CAD build for the part. Positions are in the model's coordinates, mm. A direction names the side the tool comes from. Round coordinates to 2 decimals unless told otherwise and drop trailing zeros. Loops run counter-clockwise (first coordinate to the right, second up) from the corner with the lowest first, then second, coordinate; pieces in that order, holes last.
```python
from build123d import *

# Parameters (mm, degrees)
BOSS_EXTRU_1_DEPTH      = 5
ESQUISSE2_R             = 1
ENL_V_MAT_EXTRU_1_DEPTH = 115.236596588
ESQUISSE3_R             = 3
ENL_V_MAT_EXTRU_2_DEPTH = 115.236596588
ESQUISSE4_W             = 20
ESQUISSE4_H             = 5
ENL_V_MAT_EXTRU_3_DEPTH = 115.236596588


with BuildPart() as part:
    # Esquisse1 → Boss.-Extru.1 (new body)
    with BuildSketch(Plane.XY):
        Polygon((-34, 55), (84, 55), (84, 39), (100, 39), (100, -39), (84, -39), (84, -55), (-34, -55), (-34, -39), (-50, -39), (-50, 39), (-34, 39), align=None)
    extrude(amount=-BOSS_EXTRU_1_DEPTH)

    # Esquisse2 → Enlèv. mat.-Extru.1 (cut, through all)
    with BuildSketch(Plane(origin=(0, 0, -5), x_dir=(-1, 0, 0), z_dir=(0, 0, -1))):
        with Locations((-75, -35)):
            Circle(ESQUISSE2_R)
        with Locations((-17, -35)):
            Circle(ESQUISSE2_R)
        with Locations((-75, 14)):
            Circle(ESQUISSE2_R)
        with Locations((-17, 14)):
            Circle(ESQUISSE2_R)
    extrude(amount=-ENL_V_MAT_EXTRU_1_DEPTH, mode=Mode.SUBTRACT)

    # Esquisse3 → Enlèv. mat.-Extru.2 (cut, through all)
    with BuildSketch(Plane(origin=(0, 0, -5), x_dir=(-1, 0, 0), z_dir=(0, 0, -1))):
        with Locations((-37.5, -21)):
            Circle(ESQUISSE3_R)
        with Locations((-37.5, 21)):
            Circle(ESQUISSE3_R)
        with Locations((-12.5, 21)):
            Circle(ESQUISSE3_R)
        with Locations((-12.5, -21)):
            Circle(ESQUISSE3_R)
    extrude(amount=-ENL_V_MAT_EXTRU_2_DEPTH, mode=Mode.SUBTRACT)

    # Esquisse4 → Enlèv. mat.-Extru.3 (cut, through all)
    with BuildSketch(Plane(origin=(0, 0, -5), x_dir=(-1, 0, 0), z_dir=(0, 0, -1))):
        with Locations((-55, 47.5)):
            Rectangle(ESQUISSE4_W, ESQUISSE4_H)
        with Locations((-25, 47.5)):
            Rectangle(ESQUISSE4_W, ESQUISSE4_H)
        with Locations((5, 47.5)):
            Rectangle(ESQUISSE4_W, ESQUISSE4_H)
    extrude(amount=-ENL_V_MAT_EXTRU_3_DEPTH, mode=Mode.SUBTRACT)


solid = part.part
```
Item 1: Cut at A-A, the plane x = 37.5. Give the cut face in (y, z).
Answers follow:
outline: (-55, -5) - (-24, -5) - (-24, 0) - (-55, 0) - close; (-18, -5) - (18, -5) - (18, 0) - (-18, 0) - close; (24, -5) - (55, -5) - (55, 0) - (24, 0) - close
Item 2: Cut at D-D, the plane y = -41.5. Give the cut face in (x, z).
Answers follow:
outline: (-34, -5) - (84, -5) - (84, 0) - (-34, 0) - close
Item 3: Probe line 1 (Y direction, x = 12.5, z = -1.5); line 2 (Y direction, x = 75, z = -1.6); line 3 (Y direction, x = 17, z = -2.15). List the from-to ranges inside material, lowest first.
Answers follow:
line 1: y = -55 to -24, -18 to 18, 24 to 55
line 2: y = -55 to -36, -34 to 13, 15 to 55
line 3: y = -55 to -36, -34 to 13, 15 to 45, 50 to 55
Item 4: Two-plate mould, pull along Y, no slides. Class faces 1 (the flat face through (-42, 39, -2)), 2 (the flat face through (45, 47, -3)), 3 (the flat face through (26, -55, -2)), 4 (the flat face through (84, 47, -2)): released by +Y, released by -Y, zero draft, split by the parting line, or undercut.
Answers follow:
face 1: released by +Y
face 2: undercut
face 3: released by -Y
face 4: zero draft
Item 5: 3-axis set-ups, long thin cutter, end or side, ignore diameter. For faces 5 (the flat face through (65, 47, -3)), 6 (the flat face through (100, 1, -2)), 7 (the flat face through (92, -39, -2)), 8 (the flat face through (26, 1, 0)), 9 (the flat face through (92, 39, -2)): which of +Z, -Z, +X, -X, +Y, -Y reach the whole face in a straight line?
Answers follow:
face 5: +Z, -Z
face 6: +Z, -Z, +X, +Y, -Y
face 7: +Z, -Z, +X, -Y
face 8: +Z, +X, -X, +Y, -Y
face 9: +Z, -Z, +X, +Y
Item 6: Flat gauge pins, fed straight in: P1, Ø2.5, axis at y = 48, z = -3.5, coming from the -X side; P2, Ø2.5, axis at x = 17, y = -35, coming from the -Z side; P3, Ø5, axis at x = 12.5, y = -21, coming from the -Z side. Where does each tip first touch, or does it go through?
Answers follow:
P1: stops at x = -34
P2: stops at z = -5
P3: passes through
Item 7: Cut at C-C, the plane z = -3.95. State how many separate pieces and enclosed holes the cut face has, plus the area to 3 significant figures.
Answers follow:
separate pieces: 1
enclosed holes: 11
area: 15,100 mm2
Item 8: Cut at B-B, the plane y = 21. Give the cut face in (x, z), plus the area to 3 significant figures.
Answers follow:
outline: (-50, -5) - (9.5, -5) - (9.5, 0) - (-50, 0) - close; (15.5, -5) - (34.5, -5) - (34.5, 0) - (15.5, 0) - close; (40.5, -5) - (100, -5) - (100, 0) - (40.5, 0) - close
area: 690 mm2
